```python
from build123d import *

# Parameters (mm, degrees)
EXTRUDE_1_DEPTH     = 18
SKETCH_2_W          = 32
SKETCH_2_H          = 12
CUT_EXTRUDE_1_DEPTH = 34
SKETCH_3_W          = 32
SKETCH_3_H          = 8
CUT_EXTRUDE_2_DEPTH = 34
SKETCH_4_R          = 10.5
CUT_EXTRUDE_3_DEPTH = 34
SKETCH_5_W          = 36.797591779
SKETCH_5_H          = 31.340238438
CUT_EXTRUDE_4_DEPTH = 2
SKETCH_6_W          = 48.194095428
SKETCH_6_H          = 31.947752294
CUT_EXTRUDE_5_DEPTH = 2
SKETCH_7_R          = 2
CUT_EXTRUDE_6_DEPTH = 20
SKETCH_8_W          = 5
SKETCH_8_H          = 10
CUT_EXTRUDE_7_DEPTH = 20
SKETCH_9_R          = 10.5
EXTRUDE_2_DEPTH     = 4
SKETCH_10_R         = 10.5
EXTRUDE_3_DEPTH     = 4
SKETCH_11_R         = 2
SKETCH_11_W         = 5
SKETCH_11_H         = 10
EXTRUDE_4_DEPTH     = 1
EXTRUDE_START       = 1
SKETCH_12_R         = 2
SKETCH_12_W         = 5
SKETCH_12_H         = 10
EXTRUDE_5_DEPTH     = 1
SKETCH_13_W         = 5
SKETCH_13_H         = 10
CUT_EXTRUDE_8_DEPTH = 19
FILLET_1_R          = 3


with BuildPart() as part:
    # 草图1 → 凸台-拉伸1 (new body)
    with BuildSketch(Plane.XY):
        with BuildLine():
            Line((0, 15), (38, 15))
            ThreePointArc((38, 15), (53, 0), (38, -15))
            Line((38, -15), (0, -15))
            ThreePointArc((0, -15), (-15, 0), (0, 15))
        make_face()
    extrude(amount=EXTRUDE_1_DEPTH)

    # 草图2 → 切除-拉伸1 (cut)
    with BuildSketch(Plane(origin=(0, 15, 0), x_dir=(1, 0, 0), z_dir=(0, 1, 0))):
        with Locations((1, -9)):
            Rectangle(SKETCH_2_W, SKETCH_2_H)
    extrude(amount=-CUT_EXTRUDE_1_DEPTH, mode=Mode.SUBTRACT)

    # 草图3 → 切除-拉伸2 (cut)
    with BuildSketch(Plane(origin=(0, 15, 0), x_dir=(1, 0, 0), z_dir=(0, 1, 0))):
        with Locations((37, -9)):
            Rectangle(SKETCH_3_W, SKETCH_3_H)
    extrude(amount=-CUT_EXTRUDE_2_DEPTH, mode=Mode.SUBTRACT)

    # 草图4 → 切除-拉伸3 (cut)
    with BuildSketch(Plane.XY.offset(18)):
        Circle(SKETCH_4_R)
    extrude(amount=-CUT_EXTRUDE_3_DEPTH, mode=Mode.SUBTRACT)

    # 草图5 → 切除-拉伸4 (cut)
    with BuildSketch(Plane.XY.offset(18)):
        with Locations((39.39879589, -0.670119219)):
            Rectangle(SKETCH_5_W, SKETCH_5_H)
    extrude(amount=-CUT_EXTRUDE_4_DEPTH, mode=Mode.SUBTRACT)

    # 草图6 → 切除-拉伸5 (cut)
    with BuildSketch(Plane(origin=(0, 0, 0), x_dir=(-1, 0, 0), z_dir=(0, 0, -1))):
        with Locations((-45.097047714, -0.973876147)):
            Rectangle(SKETCH_6_W, SKETCH_6_H)
    extrude(amount=-CUT_EXTRUDE_5_DEPTH, mode=Mode.SUBTRACT)

    # 草图7 → 切除-拉伸6 (cut)
    with BuildSketch(Plane(origin=(0, 0, 2), x_dir=(-1, 0, 0), z_dir=(0, 0, -1))):
        with Locations((-48, 0)):
            Circle(SKETCH_7_R)
        with Locations((-38, 10)):
            Circle(SKETCH_7_R)
        with Locations((-28, 0)):
            Circle(SKETCH_7_R)
        with Locations((-38, -10)):
            Circle(SKETCH_7_R)
    extrude(amount=-CUT_EXTRUDE_6_DEPTH, mode=Mode.SUBTRACT)

    # 草图8 → 切除-拉伸7 (cut)
    with BuildSketch(Plane(origin=(0, 0, 2), x_dir=(-1, 0, 0), z_dir=(0, 0, -1))):
        with Locations((-35.5, 0)):
            Rectangle(SKETCH_8_W, SKETCH_8_H)
    extrude(amount=-CUT_EXTRUDE_7_DEPTH, mode=Mode.SUBTRACT)

    # 草图9 → 凸台-拉伸2 (add)
    with BuildSketch(Plane(origin=(0, 0, 0), x_dir=(-1, 0, 0), z_dir=(0, 0, -1))):
        with BuildLine():
            Line((0, 15), (-21, 15))
            Line((-21, 15), (-21, -15))
            Line((-21, -15), (0, -15))
            ThreePointArc((0, -15), (15, 0), (0, 15))
        make_face()
        with Locations(Location((0, 0, 0), (0, 0, 180))):
            Circle(SKETCH_9_R, mode=Mode.SUBTRACT)
    extrude(amount=-EXTRUDE_2_DEPTH)

    # 草图10 → 凸台-拉伸3 (add)
    with BuildSketch(Plane.XY.offset(18)):
        with BuildLine():
            Line((21, -15), (21, 15))
            Line((21, 15), (0, 15))
            ThreePointArc((0, 15), (-15, 0), (0, -15))
            Line((0, -15), (21, -15))
        make_face()
        Circle(SKETCH_10_R, mode=Mode.SUBTRACT)
    extrude(amount=-EXTRUDE_3_DEPTH)

    # 草图11 → 凸台-拉伸4 (add)
    with BuildSketch(Plane.XY.offset(16)):
        with BuildLine():
            Line((21, -15), (38, -15))
            ThreePointArc((38, -15), (53, 0), (38, 15))
            Line((38, 15), (21, 15))
            Line((21, 15), (21, -15))
        make_face()
        with Locations(Location((38, 10, 0), (0, 0, 180))):
            Circle(SKETCH_11_R, mode=Mode.SUBTRACT)
        with Locations(Location((38, -10, 0), (0, 0, 180))):
            Circle(SKETCH_11_R, mode=Mode.SUBTRACT)
        with Locations(Location((28, 0, 0), (0, 0, 180))):
            Circle(SKETCH_11_R, mode=Mode.SUBTRACT)
        with Locations(Location((48, 0, 0), (0, 0, 180))):
            Circle(SKETCH_11_R, mode=Mode.SUBTRACT)
        with Locations((35.5, 0)):
            Rectangle(SKETCH_11_W, SKETCH_11_H, mode=Mode.SUBTRACT)
    extrude(amount=EXTRUDE_4_DEPTH)

    # 草图12 → 凸台-拉伸5 (add)
    with BuildSketch(Plane(origin=(0, 0, 2), x_dir=(-1, 0, 0), z_dir=(0, 0, -1)).offset(EXTRUDE_START)):
        with BuildLine():
            Line((-21, -15), (-21, 15))
            Line((-21, 15), (-38, 15))
            ThreePointArc((-38, 15), (-53, 0), (-38, -15))
            Line((-38, -15), (-21, -15))
        make_face()
        with Locations((-48, 0)):
            Circle(SKETCH_12_R, mode=Mode.SUBTRACT)
        with Locations((-38, -10)):
            Circle(SKETCH_12_R, mode=Mode.SUBTRACT)
        with Locations((-28, 0)):
            Circle(SKETCH_12_R, mode=Mode.SUBTRACT)
        with Locations((-38, 10)):
            Circle(SKETCH_12_R, mode=Mode.SUBTRACT)
        with Locations((-35.5, 0)):
            Rectangle(SKETCH_12_W, SKETCH_12_H, mode=Mode.SUBTRACT)
    extrude(amount=-EXTRUDE_5_DEPTH)

    # 草图13 → 切除-拉伸8 (cut)
    with BuildSketch(Plane.XY.offset(17)):
        with Locations((40.5, 0)):
            Rectangle(SKETCH_13_W, SKETCH_13_H)
    extrude(amount=-CUT_EXTRUDE_8_DEPTH, mode=Mode.SUBTRACT)

    # 圆角1
    fillet_1_edges = [part.edges().sort_by_distance(p)[0] for p in [
        (33, 5, 14.5),
        (33, 5, 3),
        (33, -5, 14.5),
        (33, -5, 3),
        (43, 5, 15),
        (43, 5, 3),
        (43, -5, 15),
        (43, -5, 3),
    ]]
    fillet(fillet_1_edges, radius=FILLET_1_R)


solid = part.part
```
Part model, mm, in its own coordinate system. A direction names the side the tool comes from. Round coordinates to 2 decimals unless told otherwise and drop trailing zeros. Order: outer loops, then holes, each group sorted by start corner. A loop starts at its lowest first (then second) coordinate and runs counter-clockwise, first axis right, second up. Notation, with made-up numbers: M 26.25,32 L 78.25,32 A19 ccw 78.25,54 Z; hole C 8.5,-29.5 d10. An arc over 180 degrees is marked long. Put each result on its own line as item: value. Start each with the question number.
1. Slice it at D-D on x = 4. List the corners of the cut face in (y, z), then the cut area to 3 significant figures.
2. Drop flat-ended pins along their axis: pin 1 (9 mm diameter, centred on x = 40.5, y = 3.5, fed in from +Z); pin 2 (5 mm diameter, centred on x = 38, y = -10, fed in from -Z); pin 3 (1.5 mm diameter, centred on y = 6.5, z = 8, fed in from -X). Give the stop position or say it passes through.
3. Two-plate mould, pull along Y, no slides. Class faces 6 (the face through (19, 15, 9)), 7 (the face through (38, 5, 15)), 8 (the face through (17, 0, 9)): +Y half, -Y half, draft (parallel to the pull), parting line (faces both ways), or undercut.
4. Drill centre lines: probe 1 along Y at (x, z) = (38, 3); probe 2 along Z at (x, y) = (29, -2); probe 3 along Y at (x, z) = (0, 14.95). Where is each one in solid material? Low to high. Write a range as [from, to].
5. Tool access for faces 1 (the face through (11, 0, 0)), 2 (the face through (33, 4, 13)), 3 (the face through (33, 4, 17)), 4 (the face through (11, 0, 18)), 5 (the face through (43, 0, 15)): list every direction of +Z, -Z, +X, -X, +Y, -Y with a clear straight run to the whole face (end or side of a thin tool).
6. Slice it at A-A on z = 16. List the corners of the cut face in (x, y).
7. Slice it at B-B on x = 28. List the corners of the cut face in (y, z).
8. Slice it at C-C on y = 0. State how many separate pieces and enclosed holes the cut face has, then the cut area to 3 significant figures.
Findings:
1. outline: M -15,0 L -9.71,0 L -9.71,4 L -15,4 Z; M -15,14 L -9.71,14 L -9.71,18 L -15,18 Z; M 9.71,0 L 15,0 L 15,4 L 9.71,4 Z; M 9.71,14 L 15,14 L 15,18 L 9.71,18 Z
1. area: 84.7 mm2
2. pin 1: z = 17
2. pin 2: z = 1
2. pin 3: x = 17
3. face 6: +Y half
3. face 7: undercut
3. face 8: draft
4. probe 1: [-15, -12], [-8, -5], [5, 8], [12, 15]
4. probe 2: [1, 5], [13, 17]
4. probe 3: [-15, -10.5], [10.5, 15]
5. face 1: -Z, +X, -X, +Y, -Y
5. face 2: +X, +Y, -Y
5. face 3: +Z, +X, +Y, -Y
5. face 4: +Z, +X, -X, +Y, -Y
5. face 5: +Z, -Z
6. outline: M 0,-15 L 38,-15 A15 ccw 38,15 L 0,15 A15 ccw Z; hole C 0,0 d21; hole C 28,0 d4; hole M 33,-2 A3 ccw 36,-5 L 40,-5 A3 ccw 43,-2 L 43,2 A3 ccw 40,5 L 36,5 A3 ccw 33,2 Z; hole C 38,-10 d4; hole C 38,10 d4; hole C 48,0 d4
7. outline: M -15,1 L -2,1 L -2,5 L -15,5 Z; M -15,13 L -2,13 L -2,17 L -15,17 Z; M 2,1 L 15,1 L 15,5 L 2,5 Z; M 2,13 L 15,13 L 15,17 L 2,17 Z
8. separate pieces: 9
8. enclosed holes: 0
8. area: 272 mm2
